from build123d import *

# Parameters (mm, degrees)
SKETCH_1_W          = 45
SKETCH_1_H          = 247
EXTRUDE_1_DEPTH     = 6
CUT_EXTRUDE_1_DEPTH = 249.095243808
CUT_EXTRUDE_2_DEPTH = 249.095243808
FILLET_1_R          = 2
M3X0_52_D           = 2.5
M3X0_52_DEPTH       = 8.5
M3X0_52_TIP         = 0.751075774
M3X0_51_D           = 2.5
M3X0_51_DEPTH       = 8.5
M3X0_51_TIP         = 0.751075774


with BuildPart() as part:
    # Эскиз1 → Бобышка-Вытянуть1 (new body)
    with BuildSketch(Plane(origin=(0, 0, 0), x_dir=(1, 0, 0), z_dir=(0, 1, 0))):
        with Locations((0, -123.5)):
            Rectangle(SKETCH_1_W, SKETCH_1_H)
    extrude(amount=EXTRUDE_1_DEPTH)

    # Эскиз2 → Вырез-Вытянуть1 (cut, through all)
    with BuildSketch(Plane(origin=(0, 6, 0), x_dir=(1, 0, 0), z_dir=(0, 1, 0))):
        with BuildLine():
            Line((-10.274368671, -73.5), (-10.274368671, -173.5))
            ThreePointArc((-10.274368671, -173.5), (-12.374368671, -175.6), (-14.474368671, -173.5))
            Line((-14.474368671, -173.5), (-14.474368671, -73.5))
            ThreePointArc((-14.474368671, -73.5), (-12.374368671, -71.4), (-10.274368671, -73.5))
        make_face()
        with BuildLine():
            Line((10.274368671, -73.5), (10.274368671, -173.5))
            ThreePointArc((10.274368671, -173.5), (12.374368671, -175.6), (14.474368671, -173.5))
            Line((14.474368671, -173.5), (14.474368671, -73.5))
            ThreePointArc((14.474368671, -73.5), (12.374368671, -71.4), (10.274368671, -73.5))
        make_face()
    extrude(amount=-CUT_EXTRUDE_1_DEPTH, mode=Mode.SUBTRACT)

    # Эскиз14 → Вырез-Вытянуть2 (cut, through all)
    with BuildSketch(Plane(origin=(0, 6, 0), x_dir=(1, 0, 0), z_dir=(0, 1, 0))):
        Polygon((-18.5, -10), (18.5, -10), (-18.5, -31.36195996), align=None)
        Polygon((-18.5, -35.980762114), (18.5, -14.618802154), (18.5, -57.342722074), align=None)
        Polygon((-18.5, -40.599564267), (-18.5, -67.4), (18.5, -67.4), (18.5, -61.961524227), align=None)
        Polygon((6.274368671, -71.4), (-6.274368671, -78.645016882), (-6.274368671, -71.4), align=None)
        Polygon((6.274368671, -75.730127019), (-6.274368671, -82.975143901), (6.274368671, -90.220160783), align=None)
        Polygon((-6.274368671, -87.30527092), (6.274368671, -94.550287802), (-6.274368671, -101.795304684), align=None)
        Polygon((-6.274368671, -106.125431703), (6.274368671, -98.880414821), (6.274368671, -113.370448585), align=None)
        Polygon((-6.274368671, -110.455558722), (6.274368671, -117.700575604), (-6.274368671, -124.945592486), align=None)
        Polygon((-6.274368671, -129.275719505), (6.274368671, -122.030702623), (6.274368671, -136.520736387), align=None)
        Polygon((-6.274368671, -133.605846524), (6.274368671, -140.850863406), (-6.274368671, -148.095880288), align=None)
        Polygon((-6.274368671, -152.426007307), (6.274368671, -145.180990425), (6.274368671, -159.671024189), align=None)
        Polygon((-6.274368671, -156.756134326), (6.274368671, -164.001151208), (-6.274368671, -171.24616809), align=None)
        Polygon((-6.274368671, -175.576295109), (6.274368671, -168.331278227), (6.274368671, -175.576295109), align=None)
        Polygon((-18.5, -179.6), (-18.5, -185.038475773), (18.5, -206.400435733), (18.5, -179.6), align=None)
        Polygon((-18.5, -232.381197846), (-18.5, -189.657277926), (18.5, -211.019237886), align=None)
        Polygon((18.5, -215.63804004), (18.5, -237), (-18.5, -237), align=None)
    extrude(amount=-CUT_EXTRUDE_2_DEPTH, mode=Mode.SUBTRACT)

    # Скругление1
    fillet_1_edges = [part.edges().sort_by_distance(p)[0] for p in [
        (-6.274368671, 3, 101.795304684),
        (-6.274368671, 3, 87.30527092),
        (6.274368671, 3, 94.550287802),
        (6.274368671, 3, 113.370448585),
        (-6.274368671, 3, 106.125431703),
        (6.274368671, 3, 98.880414821),
        (-6.274368671, 3, 124.945592486),
        (-6.274368671, 3, 110.455558722),
        (6.274368671, 3, 117.700575604),
        (6.274368671, 3, 136.520736387),
        (-6.274368671, 3, 129.275719505),
        (6.274368671, 3, 122.030702623),
        (-6.274368671, 3, 148.095880288),
        (-6.274368671, 3, 133.605846524),
        (6.274368671, 3, 140.850863406),
        (6.274368671, 3, 159.671024189),
        (-6.274368671, 3, 152.426007307),
        (6.274368671, 3, 145.180990425),
        (-6.274368671, 3, 171.24616809),
        (-6.274368671, 3, 156.756134326),
        (6.274368671, 3, 164.001151208),
        (6.274368671, 3, 175.576295109),
        (-6.274368671, 3, 175.576295109),
        (6.274368671, 3, 168.331278227),
        (-18.5, 3, 179.6),
        (18.5, 3, 179.6),
        (18.5, 3, 206.400435733),
        (-18.5, 3, 185.038475773),
        (18.5, 3, 211.019237886),
        (-18.5, 3, 232.381197846),
        (-18.5, 3, 189.657277926),
        (-18.5, 3, 237),
        (18.5, 3, 215.63804004),
        (18.5, 3, 237),
        (-18.5, 3, 31.36195996),
        (-18.5, 3, 10),
        (18.5, 3, 10),
        (18.5, 3, 57.342722074),
        (-18.5, 3, 35.980762114),
        (18.5, 3, 14.618802154),
        (-18.5, 3, 40.599564267),
        (18.5, 3, 61.961524227),
        (18.5, 3, 67.4),
        (-18.5, 3, 67.4),
        (-6.274368671, 3, 71.4),
        (6.274368671, 3, 71.4),
        (-6.274368671, 3, 78.645016882),
        (6.274368671, 3, 75.730127019),
        (6.274368671, 3, 90.220160783),
        (-6.274368671, 3, 82.975143901),
    ]]
    fillet(fillet_1_edges, radius=FILLET_1_R)

    # Отверстие обработанное метчиком M3x0.52
    with Locations(Plane(origin=(0, 0, 0), x_dir=(-1, 0, 0), z_dir=(0, 0, -1))):
        with Locations((-16.875, 3), (-5.625, 3), (5.625, 3), (16.875, 3)):
            Hole(M3X0_52_D / 2, depth=M3X0_52_DEPTH)
            with Locations((0, 0, -(M3X0_52_DEPTH + M3X0_52_TIP / 2))):  # 118° drill point
                Cone(0, M3X0_52_D / 2, M3X0_52_TIP, mode=Mode.SUBTRACT)

    # Отверстие обработанное метчиком M3x0.51
    with Locations(Plane.XY.offset(247)):
        with Locations((-16.875, 3), (-5.625, 3), (5.625, 3), (16.875, 3)):
            Hole(M3X0_51_D / 2, depth=M3X0_51_DEPTH)
            with Locations((0, 0, -(M3X0_51_DEPTH + M3X0_51_TIP / 2))):  # 118° drill point
                Cone(0, M3X0_51_D / 2, M3X0_51_TIP, mode=Mode.SUBTRACT)


solid = part.part
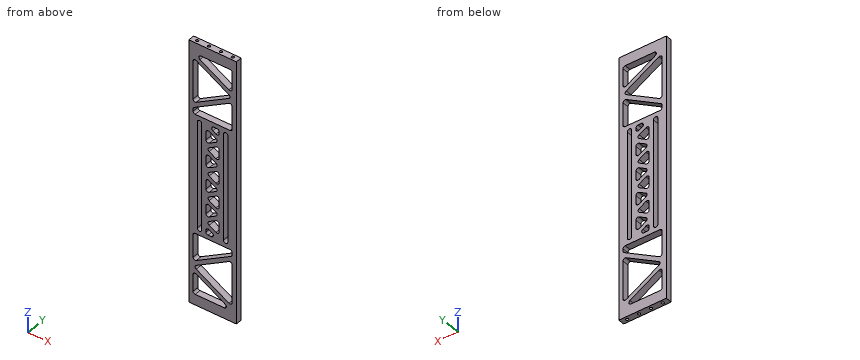
Geometry: final body of the model. Coordinates: model frame, mm. Give positions to 0.01 mm unless a question says otherwise; leave off trailing zeros. Write each loop counter-clockwise with the first axis right and the second up, starting at its lowest first coordinate (ties: lowest second). Pieces come first, ordered by that corner, then holes. Notation, with made-up numbers: (51, -17.75) -> (64, -17.75) arc R10 ccw to (64, -8.75) -> close; hole circle Ø7 at (31.5, -36.75). An arc over 180 degrees is marked (long way). Answer in a Markdown table with one row per item.
(1) Pin query (flat end, axial travel): pin 1 (1.5 mm diameter, centred on x = -5.625, y = 3, fed in from +Z); pin 2 (2 mm diameter, centred on x = 16.875, y = 3, fed in from +Z). Return the tip coordinate at first contact, or that it passes through.
Answers below:
| item | result |
|---|---|
| pin 1 | z = 238.2 |
| pin 2 | z = 238.35 |
(2) Section query A-A on z = 189. Return loops of the section in (x, y).
Answers below:
| item | result |
|---|---|
| outline | (-22.5, 0) -> (-11.64, 0) -> (-11.64, 6) -> (-22.5, 6) -> close; (18.5, 0) -> (22.5, 0) -> (22.5, 6) -> (18.5, 6) -> close |
(3) Ray query, line 1 along X through (y, z) = (4.25, 173.5); line 2 along X through (y, z) = (3, 5) (3 decimals); line 3 along Z through (x, y) = (-17, 0.5). Return the intervals inside material, ascending. Write a range as [from, to].
Answers below:
| item | result |
|---|---|
| line 1 | [-22.5, -14.47], [-10.27, -0.81], [6.27, 10.27], [14.47, 22.5] |
| line 2 | [-22.5, -18.125], [-15.625, -6.875], [-4.375, 4.375], [6.875, 15.625], [18.125, 22.5] |
| line 3 | [0, 10.06], [29.83, 42.13], [67.34, 179.66], [185.9, 191.18], [230.85, 247] |
